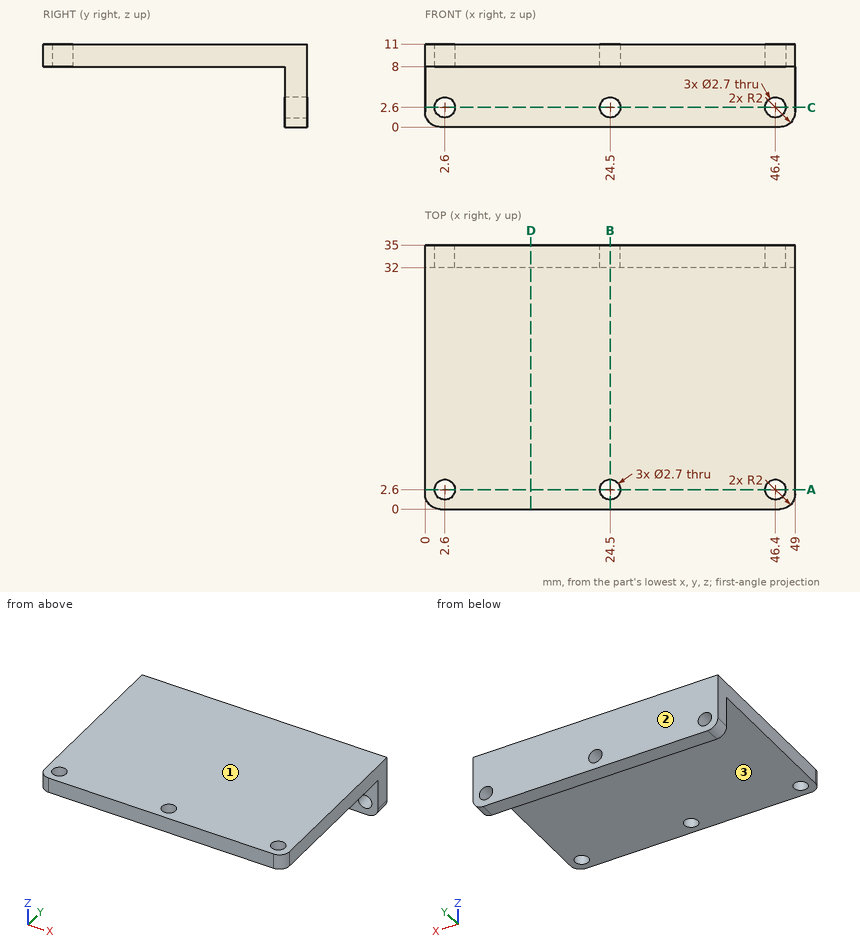
Design review of the part shown in the three views and the two pictorial views. Dimensions are in mm from the part's minimum x, y and z. Give positions to 0.01 mm unless a question says otherwise; leave off trailing zeros. Write each loop counter-clockwise with the first axis right and the second up, starting at its lowest first coordinate (ties: lowest second). Pieces come first, ordered by that corner, then holes. Notation, with made-up numbers: (22.25, -28.5) - (27.25, -28.5) arc R6 cw to (27.25, -18.5) - close; hole circle Ø5 at (71.5, 48.25). An arc over 180 degrees is marked (long way). Return JSON: item names as keys, results as strings. Group by question number.
(1) We need section C-C, the plane z = 2.6. Give the boundary of the cut face in (x, y).
(2) Mouldability with a two-part tool opening along Z and no side actions: class the marked faces 1, 2 and 3 as +Z half, -Z half, draft (parallel to the pull), parting line (faces both ways), or undercut.
(3) We need section D-D, the plane x = 14. Give the boundary of the cut face in (y, z), then the cut area to 3 significant figures.
(4) We need section A-A, the plane y = 2.6. Give the boundary of the cut face in (x, z).
(5) Insertion check: pin 1 (2 mm diameter, centred on x = 2.6, z = 2.6, fed in from +Y); pin 2 (6 mm diameter, centred on x = 40.5, z = 3.5, fed in from -Y); pin 3 (3 mm diameter, centred on x = 46.4, y = 2.6, fed in from -Z); pin 4 (4 mm diameter, centred on y = 29, z = 7, fed in from +X). Each pin has a flat end and moves straight along its axis. Give the tip position at first contact, or say it passes through.
(6) To check wall thickness, follow probe 1 along X at (y, z) = (32.75, 2.6); probe 2 along Y at (x, z) = (24.5, 10.15); probe 3 along Z at (x, y) = (10.5, 18). State the ranges of each line that lie inside material, in increasing order.
(7) We need section B-B, the plane x = 24.5. Give the boundary of the cut face in (y, z), then the cut area to 3 significant figures.
Reported:
{
 "1": {"outline": "(0, 32) - (1.25, 32) - (1.25, 35) - (0, 35) - close; (3.95, 32) - (23.15, 32) - (23.15, 35) - (3.95, 35) - close; (25.85, 32) - (45.05, 32) - (45.05, 35) - (25.85, 35) - close; (47.75, 32) - (49, 32) - (49, 35) - (47.75, 35) - close"},
 "2": {"face 1": "+Z half", "face 2": "draft", "face 3": "-Z half"},
 "3": {"outline": "(0, 8) - (32, 8) - (32, 0) - (35, 0) - (35, 11) - (0, 11) - close", "area": "129 mm2"},
 "4": {"outline": "(0, 8) - (1.25, 8) - (1.25, 11) - (0, 11) - close; (3.95, 8) - (23.15, 8) - (23.15, 11) - (3.95, 11) - close; (25.85, 8) - (45.05, 8) - (45.05, 11) - (25.85, 11) - close; (47.75, 8) - (49, 8) - (49, 11) - (47.75, 11) - close"},
 "5": {"pin 1": "passes through", "pin 2": "stops at y = 32", "pin 3": "stops at z = 8", "pin 4": "stops at x = 49"},
 "6": {"probe 1": "x = 0 to 1.25, 3.95 to 23.15, 25.85 to 45.05, 47.75 to 49", "probe 2": "y = 0 to 1.25, 3.95 to 35", "probe 3": "z = 8 to 11"},
 "7": {"outline": "(0, 8) - (1.25, 8) - (1.25, 11) - (0, 11) - close; (3.95, 8) - (32, 8) - (32, 3.95) - (35, 3.95) - (35, 11) - (3.95, 11) - close; (32, 0) - (35, 0) - (35, 1.25) - (32, 1.25) - close", "area": "113 mm2"}
}
